```python
from build123d import *

# Parameters (mm, degrees)
SKETCH1_W                                       = 100
SKETCH1_H                                       = 100
BOSS_EXTRUDE1_DEPTH                             = 2
SKETCH2_W                                       = 96.825
SKETCH2_H                                       = 96.825
SKETCH2_W_2                                     = 92.825
SKETCH2_H_2                                     = 92.825
BOSS_EXTRUDE2_DEPTH                             = 8
CSK_FOR_M2_FLAT_HEAD_MACHINE_SCREW1_D           = 2.4
CSK_FOR_M2_FLAT_HEAD_MACHINE_SCREW1_DEPTH       = 311.5
CSK_FOR_M2_FLAT_HEAD_MACHINE_SCREW1_CSINK_D     = 4.8
CSK_FOR_M2_FLAT_HEAD_MACHINE_SCREW1_CSINK_ANGLE = 90
CSK_FOR_M2_FLAT_HEAD_MACHINE_SCREW1_TIP         = 0.721032743
FILLET1_R                                       = 1
M2_CLEARANCE_HOLE1_D                            = 2.4
M2_CLEARANCE_HOLE2_D                            = 2.4


with BuildPart() as part:
    # Sketch1 → Boss-Extrude1 (new body)
    with BuildSketch(Plane.XY):
        with Locations((50, 50)):
            Rectangle(SKETCH1_W, SKETCH1_H)
        with BuildLine():
            Line((8, 16.124515497), (8, 83.875484503))
            ThreePointArc((8, 83.875484503), (8.347704775, 84.052717317), (8.691485355, 84.237446833))
            Line((8.691485355, 84.237446833), (42.928932188, 50))
            Line((42.928932188, 50), (8.691485355, 15.762553167))
            ThreePointArc((8.691485355, 15.762553167), (8.347704775, 15.947282683), (8, 16.124515497))
        make_face(mode=Mode.SUBTRACT)
        with BuildLine():
            Line((16.124515497, 92), (83.875484503, 92))
            ThreePointArc((83.875484503, 92), (84.052717317, 91.652295225), (84.237446833, 91.308514645))
            Line((84.237446833, 91.308514645), (50, 57.071067812))
            Line((50, 57.071067812), (15.762553167, 91.308514645))
            ThreePointArc((15.762553167, 91.308514645), (15.947282683, 91.652295225), (16.124515497, 92))
        make_face(mode=Mode.SUBTRACT)
        with BuildLine():
            Line((92, 83.875484503), (92, 16.124515497))
            ThreePointArc((92, 16.124515497), (91.652295225, 15.947282683), (91.308514645, 15.762553167))
            Line((91.308514645, 15.762553167), (57.071067812, 50))
            Line((57.071067812, 50), (91.308514645, 84.237446833))
            ThreePointArc((91.308514645, 84.237446833), (91.652295225, 84.052717317), (92, 83.875484503))
        make_face(mode=Mode.SUBTRACT)
        with BuildLine():
            Line((16.124515497, 8), (83.875484503, 8))
            ThreePointArc((83.875484503, 8), (84.052717317, 8.347704775), (84.237446833, 8.691485355))
            Line((84.237446833, 8.691485355), (50, 42.928932188))
            Line((50, 42.928932188), (15.762553167, 8.691485355))
            ThreePointArc((15.762553167, 8.691485355), (15.947282683, 8.347704775), (16.124515497, 8))
        make_face(mode=Mode.SUBTRACT)
    extrude(amount=BOSS_EXTRUDE1_DEPTH)

    # Sketch2 → Boss-Extrude2 (add)
    with BuildSketch(Plane.XY.offset(2)):
        with Locations((50, 50)):
            Rectangle(SKETCH2_W, SKETCH2_H)
        with Locations((50, 50)):
            Rectangle(SKETCH2_W_2, SKETCH2_H_2, mode=Mode.SUBTRACT)
    extrude(amount=BOSS_EXTRUDE2_DEPTH)

    # CSK for M2 Flat Head Machine Screw1
    with Locations(Plane.XY.offset(2)):
        with Locations((6.5, 93.5), (93.5, 93.5), (93.5, 6.5), (6.5, 6.5)):
            CounterSinkHole(CSK_FOR_M2_FLAT_HEAD_MACHINE_SCREW1_D / 2, CSK_FOR_M2_FLAT_HEAD_MACHINE_SCREW1_CSINK_D / 2, depth=CSK_FOR_M2_FLAT_HEAD_MACHINE_SCREW1_DEPTH, counter_sink_angle=CSK_FOR_M2_FLAT_HEAD_MACHINE_SCREW1_CSINK_ANGLE)
            with Locations((0, 0, -(CSK_FOR_M2_FLAT_HEAD_MACHINE_SCREW1_DEPTH + CSK_FOR_M2_FLAT_HEAD_MACHINE_SCREW1_TIP / 2))):  # 118° drill point
                Cone(0, CSK_FOR_M2_FLAT_HEAD_MACHINE_SCREW1_D / 2, CSK_FOR_M2_FLAT_HEAD_MACHINE_SCREW1_TIP, mode=Mode.SUBTRACT)

    # Fillet1
    fillet1_edges = [part.edges().sort_by_distance(p)[0] for p in [
        (0, 100, 1),
        (100, 100, 1),
        (100, 0, 1),
        (0, 0, 1),
    ]]
    fillet(fillet1_edges, radius=FILLET1_R)

    # M2 Clearance Hole1 (through all)
    with Locations(Plane.ZY.offset(-1.5875)):
        with Locations((6, 90.4125), (6, 9.5875)):
            Hole(M2_CLEARANCE_HOLE1_D / 2)

    # M2 Clearance Hole2 (through all)
    with Locations(Plane(origin=(0, 98.4125, 0), x_dir=(1, 0, 0), z_dir=(0, 1, 0))):
        with Locations((9.5875, -6), (90.4125, -6)):
            Hole(M2_CLEARANCE_HOLE2_D / 2)


solid = part.part
```
Geometry check sheet. Reference: the model listing, model coordinates, mm. A direction names the side the tool comes from. Give positions to 0.01 mm unless a question says otherwise; leave off trailing zeros. Write each loop counter-clockwise with the first axis right and the second up, starting at its lowest first coordinate (ties: lowest second). Pieces come first, ordered by that corner, then holes.
1) Section check C-C, the plane x = 18. Record the boundary of the cut face in (y, z).
2) Access from +Z, -Z, +X, -X, +Y, -Y to the whole of each face (thin tool, end or side, straight path). Record for faces 4 (the cylindrical face through (97.43, 89.24, 6.26)), 5 (the flat face through (49, 3.587, 6)), 6 (the flat face through (73.95, 66.88, 0.99)).
3) Gauge pin test, flat ends, axial feed: pin 1 (1.9 mm diameter, centred on x = 9.59, z = 6, fed in from -Y); pin 2 (6 mm diameter, centred on y = 75.5, z = 7.5, fed in from -X); pin 3 (3 mm diameter, centred on x = 81, y = 22.5, fed in from +Z); pin 4 (4 mm diameter, centred on x = 93.5, y = 6.5, fed in from +Z). Record the tip position at first contact, or that the pin passes through.
4) Section check A-A, the plane x = 6.5. Record the boundary of the cut face in (y, z).
5) Material ranges on L1, parallel to Y at x = 96.8, z = 6; L2, parallel to X at y = 6.5, z = 0.55, recorded low to high.
6) Release check for a two-part mould opening along Z. For faces 1 (the flat face through (3, 72, 10)), 2 (the cylindrical face through (2.6, 89.24, 6.26)), 3 (the cylindrical face through (94.7, 6.55, 0.39)) record: pulls with the +Z half, pulls with the -Z half, needs draft (parallel to the pull), parting line crosses it, or undercut.
7) Section check D-D, the plane y = 61. Record the boundary of the cut face in (x, z).
Computed:
1. outline: (0, 0) - (8, 0) - (8, 2) - (3.59, 2) - (3.59, 10) - (1.59, 10) - (1.59, 2) - (0, 2) - close; (10.93, 0) - (25.07, 0) - (25.07, 2) - (10.93, 2) - close; (74.93, 0) - (89.07, 0) - (89.07, 2) - (74.93, 2) - close; (92, 0) - (100, 0) - (100, 2) - (98.41, 2) - (98.41, 10) - (96.41, 10) - (96.41, 2) - (92, 2) - close
2. face 4: +X, -X
2. face 5: +Z
2. face 6: +Z, -Z
3. pin 1: passes through
3. pin 2: stops at x = 1.59
3. pin 3: stops at z = 2
3. pin 4: stops at z = 1.6
4. outline: (0, 0) - (5.3, 0) - (5.3, 0.8) - (4.1, 2) - (3.59, 2) - (3.59, 10) - (1.59, 10) - (1.59, 2) - (0, 2) - close; (7.7, 0) - (92.3, 0) - (92.3, 0.8) - (91.1, 2) - (8.9, 2) - (7.7, 0.8) - close; (94.7, 0) - (100, 0) - (100, 2) - (98.41, 2) - (98.41, 10) - (96.41, 10) - (96.41, 2) - (95.9, 2) - (94.7, 0.8) - close
5. L1: y = 1.59 to 8.39, 10.79 to 89.21, 91.61 to 98.41
5. L2: x = 0 to 5.3, 7.7 to 92.3, 94.7 to 100
6. face 1: pulls with the +Z half
6. face 2: undercut
6. face 3: needs draft
7. outline: (0, 0) - (8, 0) - (8, 2) - (3.59, 2) - (3.59, 10) - (1.59, 10) - (1.59, 2) - (0, 2) - close; (31.93, 0) - (46.07, 0) - (46.07, 2) - (31.93, 2) - close; (53.93, 0) - (68.07, 0) - (68.07, 2) - (53.93, 2) - close; (92, 0) - (100, 0) - (100, 2) - (98.41, 2) - (98.41, 10) - (96.41, 10) - (96.41, 2) - (92, 2) - close
